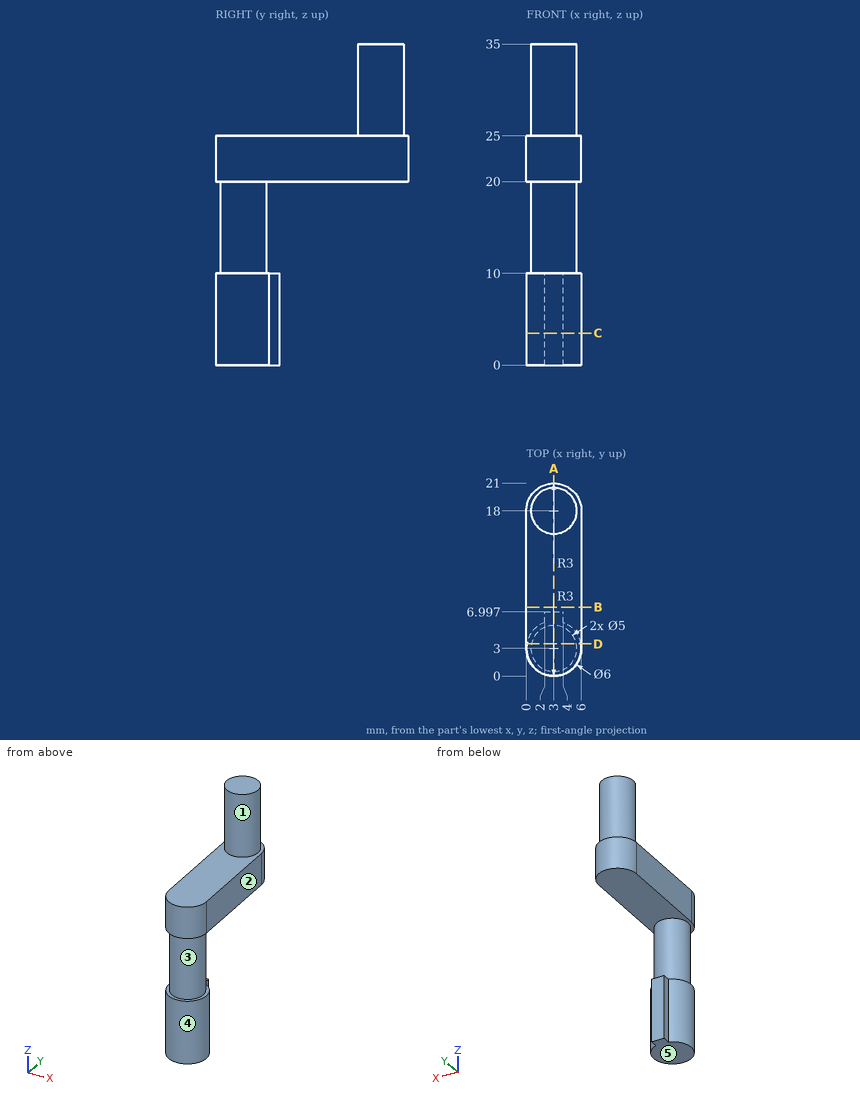
Geometry check sheet. Reference: drawing and pictorial views, mm from the part's lowest x, y, z. A direction names the side the tool comes from. Round coordinates to 2 decimals unless told otherwise and drop trailing zeros. Order: outer loops, then holes, each group sorted by start corner. A loop starts at its lowest first (then second) coordinate and runs counter-clockwise, first axis right, second up. Notation, with made-up numbers: M 47,51 L 87,51 A10 cw 87,58 Z; hole C 53,-21.75 d5. An arc over 180 degrees is marked long. Answer in a Markdown table with one row per item.
(1) Sectioned sample at C-C, the plane z = 3.5. Record the cut outline in (x, y).
Responses:
| item | result |
|---|---|
| outline | M 2,5.83 A3 ccw long 4,5.83 L 4,7 L 2,7 Z |
(2) Sectioned sample at A-A, the plane x = 3. Record the cut outline in (y, z).
Responses:
| item | result |
|---|---|
| outline | M 0,0 L 7,0 L 7,10 L 5.5,10 L 5.5,20 L 21,20 L 21,25 L 20.5,25 L 20.5,35 L 15.5,35 L 15.5,25 L 0,25 L 0,20 L 0.5,20 L 0.5,10 L 0,10 Z |
(3) Sectioned sample at B-B, the plane y = 7.5. Record the cut outline in (x, z), and give its area (3 significant figures).
Responses:
| item | result |
|---|---|
| outline | M 0,20 L 6,20 L 6,25 L 0,25 Z |
| area | 30.0 mm² |
(4) Sectioned sample at D-D, the plane y = 3.5. Record the cut outline in (x, z), and give its area (3 significant figures).
Responses:
| item | result |
|---|---|
| outline | M 0,20 L 0.55,20 L 0.55,10 L 0.04,10 L 0.04,0 L 5.96,0 L 5.96,10 L 5.45,10 L 5.45,20 L 6,20 L 6,25 L 0,25 Z |
| area | 138 mm² |
(5) Draft check along Z on the marked faces 3, 4 and 5. Enter one of: released by +Z, released by -Z, zero draft, split by the parting line, or undercut.
Responses:
| item | result |
|---|---|
| face 3 | undercut |
| face 4 | zero draft |
| face 5 | released by -Z |
(6) Scan lines: probe 1 along Z at (x, y) = (0.5, 1.75); probe 2 along Z at (x, y) = (2.25, 12.5); probe 3 along Z at (x, y) = (0.75, 18.5). Record each from-to range of solid material in increasing order. Write a range as from..to.
Responses:
| item | result |
|---|---|
| probe 1 | z = 0..10, 20..25 |
| probe 2 | z = 20..25 |
| probe 3 | z = 20..35 |
(7) Go/stop test with flat-tipped pins: P1, Ø3, axis at x = 4.5, y = 6, coming from the +Z side; P2, Ø0.9, axis at y = 6.5, z = 5.5, coming from the +X side; P3, Ø1, axis at x = 3, z = 7, coming from the +Y side; P4, Ø3, axis at x = 1, y = 4.5, coming from the -Z side. Record where each tip stops, or that it passes through.
Responses:
| item | result |
|---|---|
| P1 | stops at z = 25 |
| P2 | stops at x = 4 |
| P3 | stops at y = 7 |
| P4 | stops at z = 0 |
(8) Tool access check on the marked faces 1 and 2. Record the directions out of +Z, -Z, +X, -X, +Y, -Y that give a thin tool (end or side, any length) a straight path to the whole face; none if there is none.
Responses:
| item | result |
|---|---|
| face 1 | +Z |
| face 2 | +Z, -Z, +X, +Y, -Y |
